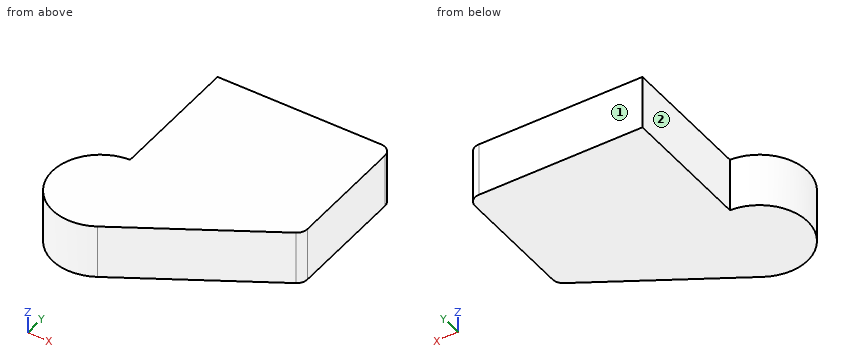
```python
from build123d import *

# Parameters (mm, degrees)
F1_DEPTH = 25.4
F2_R     = 5.08
F3_R     = 5.08


with BuildPart() as f1:
    # F0 (on Top) → F1 (new body)
    with BuildSketch(Plane.XY):
        with BuildLine():
            Line((-36.114874, 41.076776), (-36.114874, -21.335141))
            ThreePointArc((-36.114874, -21.335141), (-56.840589, -50.317389), (-23.684892, -63.364446))
            Line((-23.684892, -63.364446), (46.034314, -22.190897))
            Line((46.034314, -22.190897), (46.034314, 41.076776))
            Line((46.034314, 41.076776), (-36.114874, 41.076776))
        make_face()
    extrude(amount=F1_DEPTH)

    # F2
    f2_edges = [f1.edges().sort_by_distance(p)[0] for p in [
        (46.034314, -22.190897, 12.7),
    ]]
    fillet(f2_edges, radius=F2_R)

    # F3
    f3_edges = [f1.edges().sort_by_distance(p)[0] for p in [
        (46.034314, 41.076776, 12.7),
    ]]
    fillet(f3_edges, radius=F3_R)


solid = f1.part
```
Work out the finished part from the listing and answer in its coordinate system (mm). Face numbers are marked on the shaded views. A direction names the side the tool comes from. Give positions to 0.01 mm unless a question says otherwise; leave off trailing zeros. Loops run counter-clockwise (first coordinate to the right, second up) from the corner with the lowest first, then second, coordinate; pieces in that order, holes last. Notation, with made-up numbers: (-36.5, 23.25) -> (-25.5, 23.25) arc R26 ccw to (-25.5, 52.25) -> close; hole circle Ø7 at (0.25, 70). An arc over 180 degrees is marked (long way). One line per question, with ' | ' between items. Start each with the question number.
1) Section B-B, the plane y = 5 is taken. Determine the outline of the cut face in (x, z).
2) Straight lines are drawn through the part: L1, parallel to X at y = -6, z = 5.75; L2, parallel to X at y = -46, z = 23.25; L3, parallel to Y at x = 7.5, z = 8. For each, find the intervals that lie inside material, in ascending order.
3) Section C-C, the plane x = -15.5 is taken. Determine the outline of the cut face in (y, z).
4) Section A-A, the plane z = 9 is taken. Determine the outline of the cut face in (x, y), then the cut area to 3 significant figures.
5) For the marked faces 1 and 2, determine the directions among +Z, -Z, +X, -X, +Y, -Y from which every point of the face is accessible in a straight line to the end or side of a thin tool.
6) Each of these flat-tipped pins is pushed along its axis until it touches: pin 1 (1 mm diameter, centred on y = -26.5, z = 7.5, fed in from -X); pin 2 (12 mm diameter, centred on x = -42.5, z = 16, fed in from -Y); pin 3 (4 mm diameter, centred on y = -39, z = 5.5, fed in from -X). Where does it stop, or does it pass through?
Resolved:
1) outline: (-36.11, 0) -> (46.03, 0) -> (46.03, 25.4) -> (-36.11, 25.4) -> close
2) L1: -36.11 to 46.03 | L2: -57.67 to 5.72 | L3: -44.95 to 41.08
3) outline: (-58.53, 0) -> (41.08, 0) -> (41.08, 25.4) -> (-58.53, 25.4) -> close
4) outline: (-36.11, -21.34) arc R22.59 ccw (long way) to (-23.68, -63.36) -> (43.54, -23.67) arc R5.08 ccw to (46.03, -19.29) -> (46.03, 36) arc R5.08 ccw to (40.95, 41.08) -> (-36.11, 41.08) -> close | area: 7,920 mm2
5) face 1: +Z, -Z, +X, -X, +Y | face 2: +Z, -Z, -X, +Y
6) pin 1: x = -50.16 | pin 2: y = -66.46 | pin 3: x = -57.58
